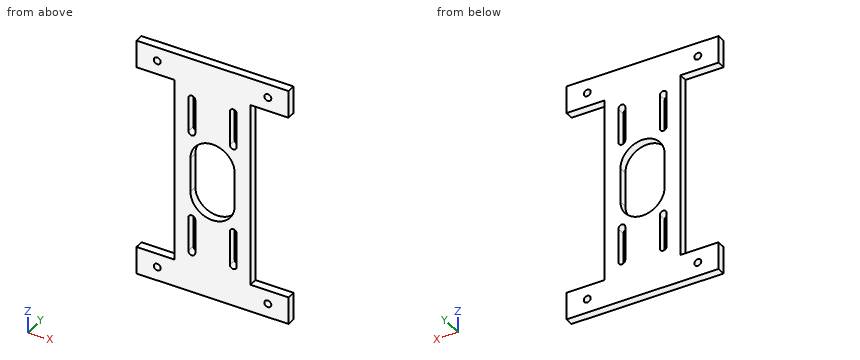
from build123d import *

# Parameters (mm, degrees)
SKETCH1_W           = 55
SKETCH1_H           = 135
SKETCH1_W_2         = 110
SKETCH1_H_2         = 20
SKETCH1_R           = 2.5
BOSS_EXTRUDE1_DEPTH = 6


with BuildPart() as part:
    # Sketch1 → Boss-Extrude1 (new body)
    with BuildSketch(Plane(origin=(0, 0, 0), x_dir=(1, 0, 0), z_dir=(0, 1, 0))):
        Rectangle(SKETCH1_W, SKETCH1_H)
        with BuildLine():
            Line((-16, -12.5), (-16, 12.5))
            ThreePointArc((-16, 12.5), (0, 28.5), (16, 12.5))
            Line((16, 12.5), (16, -12.5))
            ThreePointArc((16, -12.5), (0, -28.5), (-16, -12.5))
        make_face(mode=Mode.SUBTRACT)
        with BuildLine():
            Line((-12.5, -32.5), (-12.5, -57.5))
            ThreePointArc((-12.5, -57.5), (-15, -60), (-17.5, -57.5))
            Line((-17.5, -57.5), (-17.5, -32.5))
            ThreePointArc((-17.5, -32.5), (-15, -30), (-12.5, -32.5))
        make_face(mode=Mode.SUBTRACT)
        with BuildLine():
            Line((-12.5, 32.5), (-12.5, 57.5))
            ThreePointArc((-12.5, 57.5), (-15, 60), (-17.5, 57.5))
            Line((-17.5, 57.5), (-17.5, 32.5))
            ThreePointArc((-17.5, 32.5), (-15, 30), (-12.5, 32.5))
        make_face(mode=Mode.SUBTRACT)
        with BuildLine():
            Line((12.5, -32.5), (12.5, -57.5))
            ThreePointArc((12.5, -57.5), (15, -60), (17.5, -57.5))
            Line((17.5, -57.5), (17.5, -32.5))
            ThreePointArc((17.5, -32.5), (15, -30), (12.5, -32.5))
        make_face(mode=Mode.SUBTRACT)
        with BuildLine():
            Line((12.5, 32.5), (12.5, 57.5))
            ThreePointArc((12.5, 57.5), (15, 60), (17.5, 57.5))
            Line((17.5, 57.5), (17.5, 32.5))
            ThreePointArc((17.5, 32.5), (15, 30), (12.5, 32.5))
        make_face(mode=Mode.SUBTRACT)
        with Locations((0, -77.5)):
            Rectangle(SKETCH1_W_2, SKETCH1_H_2)
        with Locations((-40, -77.5)):
            Circle(SKETCH1_R, mode=Mode.SUBTRACT)
        with Locations((40, -77.5)):
            Circle(SKETCH1_R, mode=Mode.SUBTRACT)
        with Locations((0, 77.5)):
            Rectangle(SKETCH1_W_2, SKETCH1_H_2)
        with Locations((40, 77.5)):
            Circle(SKETCH1_R, mode=Mode.SUBTRACT)
        with Locations((-40, 77.5)):
            Circle(SKETCH1_R, mode=Mode.SUBTRACT)
    extrude(amount=BOSS_EXTRUDE1_DEPTH)


solid = part.part
The listing builds one solid part. Answer for the finished solid, in the listing's coordinates (mm). Give positions to 0.01 mm unless a question says otherwise; leave off trailing zeros. Loops run counter-clockwise (first coordinate to the right, second up) from the corner with the lowest first, then second, coordinate; pieces in that order, holes last. Notation, with made-up numbers: (-17.75, 4) - (-12.75, 4) arc R16 cw to (-12.75, 19) - close; hole circle Ø9 at (82, -39.5). An arc over 180 degrees is marked (long way). Answer as a JSON object with one key per item and string values.
1. Find the intervals of material crossed by L1, parallel to Z at x = 40, y = 2.95; L2, parallel to X at y = 3.9, z = 77.5; L3, parallel to X at y = 4.25, z = -34.5, in increasing order. Write a range as [from, to].
Determined:
{"L1": "[-87.5, -80], [-75, -67.5], [67.5, 75], [80, 87.5]", "L2": "[-55, -42.5], [-37.5, 37.5], [42.5, 55]", "L3": "[-27.5, -17.5], [-12.5, 12.5], [17.5, 27.5]"}
2. A cutting plane is placed at D-D (z = 4). Write down the section's boundary in (x, y).
Determined:
{"outline": "(-27.5, 0) - (-16, 0) - (-16, 6) - (-27.5, 6) - close; (16, 0) - (27.5, 0) - (27.5, 6) - (16, 6) - close"}
3. A cutting plane is placed at C-C (x = -40). Write down the section's boundary in (y, z), then the cut area to 3 significant figures.
Determined:
{"outline": "(0, -87.5) - (6, -87.5) - (6, -80) - (0, -80) - close; (0, -75) - (6, -75) - (6, -67.5) - (0, -67.5) - close; (0, 67.5) - (6, 67.5) - (6, 75) - (0, 75) - close; (0, 80) - (6, 80) - (6, 87.5) - (0, 87.5) - close", "area": "180 mm²"}
4. A cutting plane is placed at A-A (z = -37.5). Write down the section's boundary in (x, y).
Determined:
{"outline": "(-27.5, 0) - (-17.5, 0) - (-17.5, 6) - (-27.5, 6) - close; (-12.5, 0) - (12.5, 0) - (12.5, 6) - (-12.5, 6) - close; (17.5, 0) - (27.5, 0) - (27.5, 6) - (17.5, 6) - close"}
5. Flat-ended cylindrical pins translate along their axes: pin 1 Ø3 at (y, z) = (3, -0.5) entering from +X; pin 2 Ø1.8 at (y, z) = (4, 50.5) entering from -X. Find the tip coordinate at first contact, or state that the pin passes through.
Determined:
{"pin 1": "x = 27.5", "pin 2": "x = -27.5"}
6. A cutting plane is placed at B-B (x = 33). Write down the section's boundary in (y, z).
Determined:
{"outline": "(0, -87.5) - (6, -87.5) - (6, -67.5) - (0, -67.5) - close; (0, 67.5) - (6, 67.5) - (6, 87.5) - (0, 87.5) - close"}
